Autodesk Inventor part; units mm, degrees
ref_plane "YZ Plane" through (0, 0, 0) normal (1, 0, 0) x (0, 1, 0)
ref_plane "XZ Plane" through (0, 0, 0) normal (0, 1, 0) x (-1, 0, 0)
ref_plane "XY Plane" through (0, 0, 0) normal (0, 0, 1) x (1, 0, 0)
sketch "Sketch90" plane through (0, 0, 0) normal (0, 0, 1) x (1, 0, 0)
  circle A0 centre (0, 0) radius 2.2
  circle A1 centre (0, 0) radius 6
  dimension "d450" = 4.4
  dimension "d451" = 12
extrude "Extrusion69" add sketch "Sketch90" along normal blind 4
sketch "Sketch91" plane through (0, 0, 0) normal (1, 0, 0) x (0, 1, 0)
  line L0 (6, 0) -> (6, 4)
  line L1 (6, 4) -> (8, 4)
  line L2 (6, 0) -> (8, 0)
  line L3 (8, 4) -> (6, 2)
  line L4 (8, 0) -> (6, 2)
  line L5 (0, 0) -> (0, -8)
  line L6 (2.2, 0) -> (-2.2, 0)
  line L7 (-6, 0) -> (6, 0)
  line L8 (-2.2, 4) -> (2.2, 4)
  line L9 (6, 4) -> (-6, 4)
  line L10 (-2.2, 4) -> (2.2, 4)
  line L11 (2.2, 0) -> (-2.2, 0)
  line L12 (2.2, 0) -> (-2.2, 0)
  line L13 (2.2, 0) -> (2.2, 4)
  line L14 (2.2, 0) -> (4.2, 0)
  line L15 (4.2, 0) -> (4.2, 0)
  line L16 (3.2, -1) -> (2.2, -1)
  line L17 (2.2, -1) -> (2.2, 0)
  line L18 (-2.2, 4) -> (2.2, 4)
  line L19 (2.2, 4) -> (4.2, 4)
  line L20 (4.2, 4) -> (4.2, 4)
  line L21 (3.2, 5) -> (2.2, 5)
  line L22 (2.2, 5) -> (2.2, 4)
  line L23 (4.2, 0) -> (3.2, -1)
  line L24 (4.2, 4) -> (3.2, 5)
  point P0 (4.2, -1)
  point P1 (4.2, 5)
  dimension "d454" = 2
  dimension "d456" = 2
  dimension "d457" = 1
  dimension "d458" = 1
  dimension "d459" = 1
  dimension "d460" = 1
  dimension "d461" = 1
  dimension "d462" = 1
revolve "Revolution9" add sketch "Sketch91" angle 360 about axis through (0, 0, 0) along (0, 0, -1) contours L0 L4 L2 | L0 L1 L3 | L23 L16 L17 L7 | L9 L22 L21 L24
properties part number "wheel-4-12"
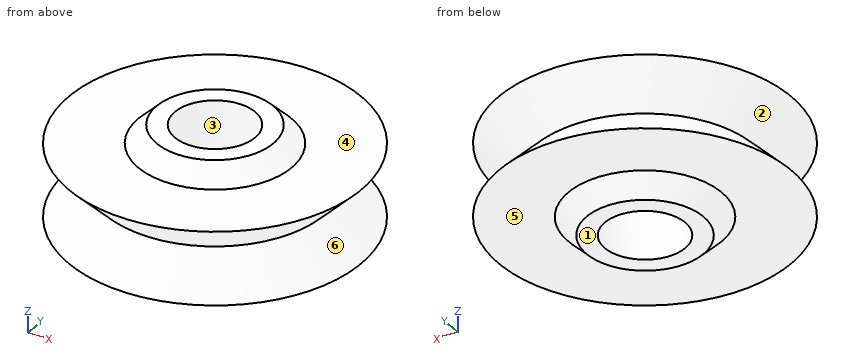
Verification items for the finished model (mm, model axes). Face numbers are marked on the shaded views. A direction names the side the tool comes from. Coordinates: 2 decimals unless noted, no trailing zeros. Order: outer loops, then holes, each group sorted by start corner. A loop starts at its lowest first (then second) coordinate and runs counter-clockwise, first axis right, second up. Notation, with made-up numbers: M 15,57.25 L 24,57.25 A16 cw 24,70.25 Z; hole C -28.75,66.25 d10. An arc over 180 degrees is marked long. One line per item, written item: value. Start each with the question number.
Item 1: Scan lines: probe 1 along X at (y, z) = (0, 1.3); probe 2 along Y at (x, z) = (-1.25, 3.1); probe 3 along Z at (x, y) = (-2.25, 4.75). Record each from-to range of solid material in increasing order.
Item 2: Gauge pin test, flat ends, axial feed: pin 1 (2 mm diameter, centred on x = -3, z = 1.5, fed in from +Y); pin 2 (1.5 mm diameter, centred on x = 5.5, y = 2, fed in from -Z). Record the tip position at first contact, or that the pin passes through.
Item 3: Access from +Z, -Z, +X, -X, +Y, -Y to the whole of each face (thin tool, end or side, straight path). Record for the marked faces 4, 5 and 6.
Item 4: Sectioned sample at A-A (z = 0.35). Enter the section's corners in (x, y).
Item 5: Mould release check, pull along X, two halves, no side actions. Record for the marked faces 1, 2 and 3: released by +X, released by -X, zero draft, split by the parting line, or undercut.
Conclusion:
1. probe 1: x = -6.7 to -2.2, 2.2 to 6.7
1. probe 2: y = -6.99 to -1.81, 1.81 to 6.99
1. probe 3: z = 0 to 4
2. pin 1: stops at y = 6.95
2. pin 2: stops at z = 0
3. face 4: +Z
3. face 5: -Z
3. face 6: none
4. outline: C 0,0 d15.3; hole C 0,0 d4.4
5. face 1: zero draft
5. face 2: split by the parting line
5. face 3: undercut
